Autodesk Inventor part; units mm, degrees
ref_plane "YZ Plane" through (0, 0, 0) normal (1, 0, 0) x (0, 1, 0)
ref_plane "XZ Plane" through (0, 0, 0) normal (0, 1, 0) x (-1, 0, 0)
ref_plane "XY Plane" through (0, 0, 0) normal (0, 0, 1) x (1, 0, 0)
sketch "Sketch1" plane through (0, 0, 0) normal (0, 0, 1) x (1, 0, 0)
  line L0 (-27.5, 27.5) -> (27.5, 27.5)
  line L1 (27.5, 27.5) -> (27.5, -27.5)
  line L2 (27.5, -27.5) -> (-27.5, -27.5)
  line L3 (-27.5, -27.5) -> (-27.5, 27.5)
  line L4 (-27.5, 27.5) -> (27.5, -27.5) construction
  line L5 (27.5, 27.5) -> (-27.5, -27.5) construction
  point P0 (0, 0)
  dimension "d0" = 55
  dimension "d1" = 55
extrude "Extrusion1" add sketch "Sketch1" along normal blind 25
sketch "Sketch2" plane through (0, 0, 25) normal (0, 0, 1) x (1, 0, 0)
  line L0 (27.5, 39) -> (-27.5, 39)
  line L1 (-27.5, 39) -> (-27.5, -39)
  line L2 (-27.5, -39) -> (27.5, -39)
  line L3 (27.5, -39) -> (27.5, 39)
  line L4 (27.5, 39) -> (-27.5, -39) construction
  line L5 (-27.5, 39) -> (27.5, -39) construction
  point P0 (0, 0)
  dimension "d4" = 55
  dimension "d5" = 78
extrude "Extrusion2" add sketch "Sketch2" along normal blind 11.5
sketch "Sketch3" plane through (0, 0, 36.5) normal (0, 0, 1) x (1, 0, 0)
  circle A0 centre (0, 0) radius 13
extrude "Extrusion3" cut sketch "Sketch3" against normal through all
sketch "Sketch4" plane through (0, 0, 36.5) normal (0, 0, 1) x (1, 0, 0)
  line L0 (27.5, -39) -> (27.5, 39)
  line L1 (27.5, 39) -> (-27.5, 39)
  line L2 (-27.5, 39) -> (-27.5, -39)
  line L3 (-27.5, -39) -> (27.5, -39)
  point P0 (0, 0)
  point P1 (22.5, 33.5)
  point P2 (22.5, -33.5)
  point P3 (7.5, 33.5)
  point P4 (7.5, -33.5)
  point P5 (-7.5, 33.5)
  point P6 (-7.5, -33.5)
  point P7 (-22.5, 33.5)
  point P8 (-22.5, -33.5)
  dimension "d10" = 5
  dimension "d11" = 5.5
  dimension "d14" = 67
  dimension "d17" = 15
  dimension "d20" = 5
  dimension "d21" = 5.5
hole "Hole1" at (22.5, 33.5, 36.5) at (22.5, -33.5, 36.5) at (7.5, 33.5, 36.5) at (7.5, -33.5, 36.5) at (-7.5, 33.5, 36.5) at (-7.5, -33.5, 36.5) at (-22.5, 33.5, 36.5) at (-22.5, -33.5, 36.5) direction (0, 0, -1) diameter 6.5 end through all
sketch "Sketch6" plane through (0, 0, 0) normal (0, 0, -1) x (-1, 0, 0)
  circle A0 centre (0, 0) radius 20
  dimension "d40" = 40
extrude "Extrusion5" cut sketch "Sketch6" against normal blind 25
chamfer "Chamfer1" distance 6.5 angle 45 4 edges at (27.5, -27.5, 12.5) (-27.5, -27.5, 12.5) (-27.5, 27.5, 12.5) (27.5, 27.5, 12.5)
chamfer "Chamfer2" distance 2 angle 45 4 edges at (27.5, -39, 30.75) (-27.5, -39, 30.75) (27.5, 39, 30.75) (-27.5, 39, 30.75)
sketch "Sketch5" plane through (-21, -27.5, 0) normal (0, -1, 0) x (1, 0, 0)
  line L0 (42, 0) -> (0, 0)
  line L1 (0, 25) -> (42, 25)
  line L2 (8.5, 0) -> (33.5, 0)
  line L3 (33.5, 0) -> (33.5, 25)
  line L4 (33.5, 25) -> (8.5, 25)
  line L5 (8.5, 25) -> (8.5, 0)
  point P0 (21, 0)
  dimension "d35" = 25
  dimension "d36" = 12.5
  dimension "d37" = 12.5
extrude "Extrusion4" cut sketch "Sketch5" against normal blind 28
equation "\"d4\" = d0"
properties part number "Y-servo-flange" material "Aluminum 6061-AHC"
CAD build for the part. Positions are in the model's coordinates, mm. A direction names the side the tool comes from. Coordinates: 2 decimals unless noted, no trailing zeros. Write each loop counter-clockwise with the first axis right and the second up, starting at its lowest first coordinate (ties: lowest second). Pieces come first, ordered by that corner, then holes. Notation, with made-up numbers: M 76,-34 L 104,-34 A16 ccw 104,-23 Z; hole C 50,15 d2. An arc over 180 degrees is marked long. Return JSON: item names as keys, results as strings.
Item 1: Slice it at D-D, the plane z = 30. State how many separate pieces and enclosed holes the cut face has, and give its area (3 significant figures).
Findings below:
{"separate pieces": "1", "enclosed holes": "9", "area": "3,490 mm2"}
Item 2: Slice it at A-A, the plane y = 33.5. Write the cut outline in (x, z).
Findings below:
{"outline": "M -27.5,25 L -25.75,25 L -25.75,36.5 L -27.5,36.5 Z; M -19.25,25 L -10.75,25 L -10.75,36.5 L -19.25,36.5 Z; M -4.25,25 L 4.25,25 L 4.25,36.5 L -4.25,36.5 Z; M 10.75,25 L 19.25,25 L 19.25,36.5 L 10.75,36.5 Z; M 25.75,25 L 27.5,25 L 27.5,36.5 L 25.75,36.5 Z"}
Item 3: Drop flat-ended pins along their axis: pin 1 Ø1 at (x, z) = (-0.5, 20.5) entering from +Y; pin 2 Ø10.5 at (x, y) = (-7.5, 33.5) entering from -Z; pin 3 Ø9.5 at (x, z) = (-15.5, 14.5) entering from -Y. Give the stop position or say it passes through.
Findings below:
{"pin 1": "stops at y = 27.5", "pin 2": "stops at z = 25", "pin 3": "stops at y = -27.5"}
Item 4: Slice it at C-C, the plane x = 22.5. Write the cut outline in (y, z).
Findings below:
{"outline": "M -39,25 L -36.75,25 L -36.75,36.5 L -39,36.5 Z; M -30.25,25 L -26,25 L -26,0 L 26,0 L 26,25 L 30.25,25 L 30.25,36.5 L -30.25,36.5 Z; M 36.75,25 L 39,25 L 39,36.5 L 36.75,36.5 Z"}
Item 5: Probe line 1 (X direction, y = 33.5, z = 28.5); line 2 (Y direction, x = -22.5, z = 31); line 3 (Y direction, x = -7.5, z = 29.75). List the from-to ranges inside material, lowest first. Write a range as from..to.
Findings below:
{"line 1": "x = -27.5..-25.75, -19.25..-10.75, -4.25..4.25, 10.75..19.25, 25.75..27.5", "line 2": "y = -39..-36.75, -30.25..30.25, 36.75..39", "line 3": "y = -39..-36.75, -30.25..-10.62, 10.62..30.25, 36.75..39"}
Item 6: Slice it at B-B, the plane x = 0. Write the cut outline in (y, z), and give its area (4 significant figures).
Findings below:
{"outline": "M -39,25 L -13,25 L -13,36.5 L -39,36.5 Z; M 13,25 L 20,25 L 20,0 L 27.5,0 L 27.5,25 L 39,25 L 39,36.5 L 13,36.5 Z", "area": "785.5 mm2"}
Item 7: Which spindle directions (+Z, -Z, +X, -X, +Y, -Y) get a long thin tool onto all of the face, cutting with end or side? Do faces 1 (the flat face through (24.2, -24.3, 12.7)), 2 (the flat face through (-24.3, 24.2, 12.3)), 3 (the flat face through (24.2, 24.3, 12.3)), 4 (the flat face through (-17, -27.5, 12)). Say none if no direction does.
Findings below:
{"face 1": "-Z, +X, -Y", "face 2": "-Z, -X, +Y", "face 3": "-Z, +X, +Y", "face 4": "-Z, +X, -X, -Y"}
Item 8: Two-plate mould, pull along Y, no slides. Class faces 5 (the flat face through (12.5, -22, 12)), 6 (the flat face through (0, -16, 25)), 7 (the flat face through (-26.5, -38, 30.7)): +Y half, -Y half, draft (parallel to the pull), parting line (faces both ways), or undercut.
Findings below:
{"face 5": "draft", "face 6": "undercut", "face 7": "-Y half"}
